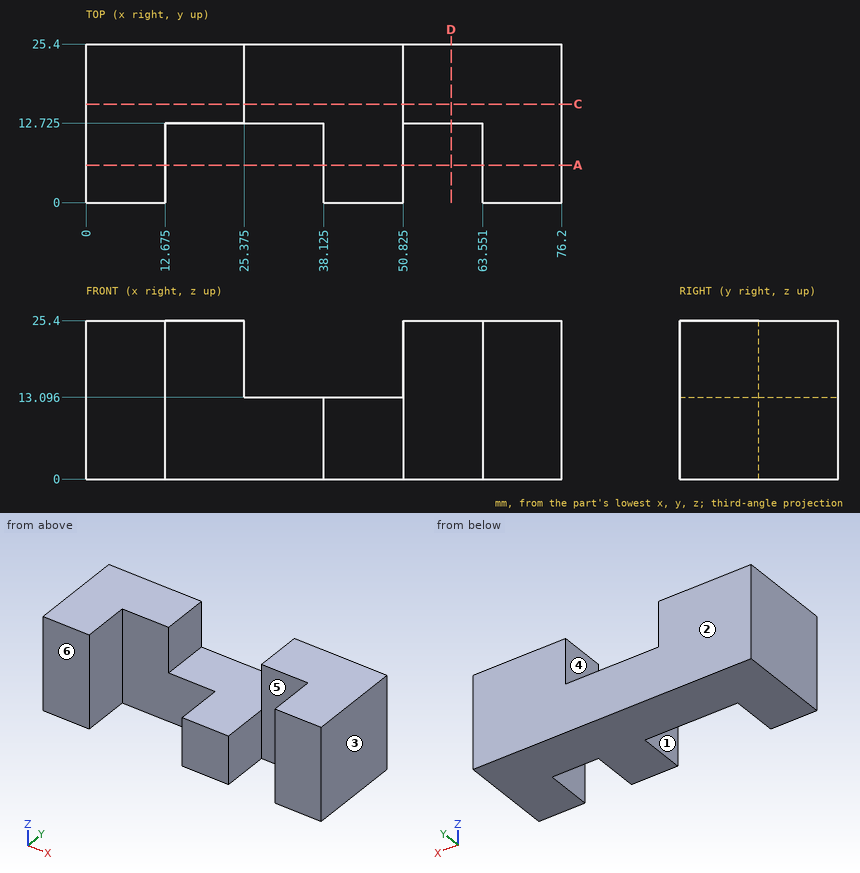
Verification items for this drawing (mm, ordinates from the low corner). A direction names the side the tool comes from. Give positions to 0.01 mm unless a question says otherwise; leave off trailing zeros. Order: outer loops, then holes, each group sorted by start corner. A loop starts at its lowest first (then second) coordinate and runs counter-clockwise, first axis right, second up.
1) Cross-section at C-C (y = 15.75). Record the boundary of the cut face in (x, z) (1 decimal).
Results are:
outline: (0, 0) - (76.2, 0) - (76.2, 25.4) - (50.8, 25.4) - (50.8, 13.1) - (25.4, 13.1) - (25.4, 25.4) - (0, 25.4) - close
2) Gauge pin test, flat end, axial feed: pin 1 (2 mm diameter, centred on x = 27, z = 10.5, fed in from -Y) (1 decimal). Record the tip position at first contact, or that the pin passes through.
Results are:
pin 1: stops at y = 12.7
3) Draft check along X on the marked faces 1, 2 and 3. Enter one of: released by +X, released by -X, zero draft, split by the parting line, or undercut.
Results are:
face 1: undercut
face 2: zero draft
face 3: released by +X
4) Cross-section at A-A (y = 6). Give the number of separate pieces and of enclosed holes in the cut face.
Results are:
separate pieces: 3
enclosed holes: 0
5) Material ranges on probe 1 along X at (y, z) = (22.75, 18.5) (1 decimal); probe 2 along Y at (x, z) = (62.5, 6.5) (1 decimal); probe 3 along Z at (x, y) = (26.5, 17) (1 decimal), recorded low to high.
Results are:
probe 1: x = 0 to 25.4, 50.8 to 76.2
probe 2: y = 12.7 to 25.4
probe 3: z = 0 to 13.1
6) Tool access check on the marked faces 4, 5 and 6. Record the directions out of +Z, -Z, +X, -X, +Y, -Y that give a thin tool (end or side, any length) a straight path to the whole face; none if there is none.
Results are:
face 4: +Z, +Y, -Y
face 5: +Z, -Z, -Y
face 6: +Z, -Z, +X, -X, -Y
7) Cross-section at D-D (x = 58.5). Record the boundary of the cut face in (y, z) (1 decimal), then the cut area to 3 significant figures.
Results are:
outline: (12.7, 0) - (25.4, 0) - (25.4, 25.4) - (12.7, 25.4) - close
area: 322 mm2
